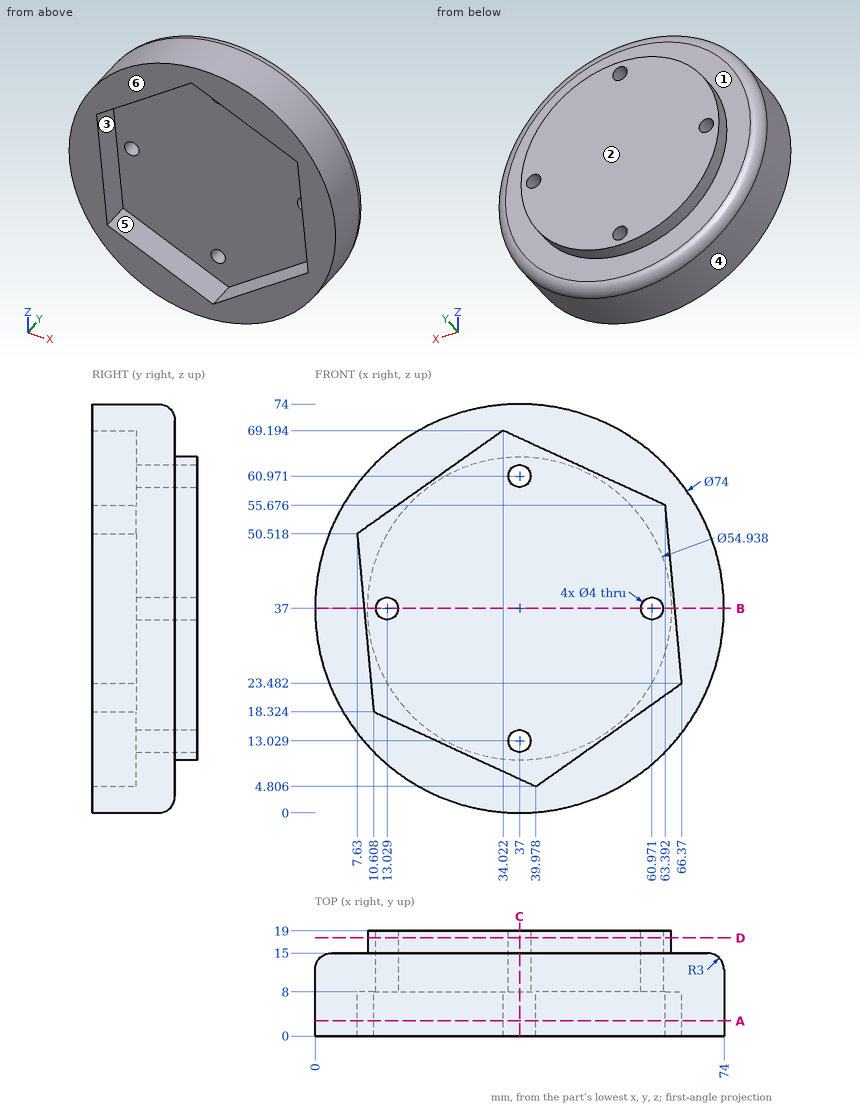
Check sheet for the drawn part. Datum: minimum x, y, z corner. Units: mm. A direction names the side the tool comes from. Round coordinates to 2 decimals unless told otherwise and drop trailing zeros. Order: outer loops, then holes, each group sorted by start corner. A loop starts at its lowest first (then second) coordinate and runs counter-clockwise, first axis right, second up.
(1) Go/stop test with flat-tipped pins: P1, Ø3, axis at y = 6, z = 16, coming from the -X side (1 decimal); P2, Ø10, axis at x = 11, y = 3, coming from the -Z side; P3, Ø17.5, axis at x = 25.5, z = 24, coming from the -Y side; P4, Ø3, axis at x = 13.029, z = 37, coming from the -Y side. Record where each tip stops, or that it passes through.
(2) Cross-section at D-D, the plane y = 17.75. Enter the section's corners in (x, z), and give its area (3 significant figures).
(3) Draft check along X on the marked faces 4, 5 and 6. Enter one of: pulls with the +X half, pulls with the -X half, needs draft (parallel to the pull), parting line crosses it, or undercut.
(4) Cross-section at B-B, the plane z = 37. Enter the section's corners in (x, y), and give its area (3 significant figures).
(5) Cross-section at A-A, the plane y = 2.75. Enter the section's corners in (x, z), and give its area (4 significant figures).
(6) Scan lines: probe 1 along Z at (x, y) = (37, 15.5); probe 2 along Z at (x, y) = (37, 14) (1 decimal); probe 3 along Y at (x, z) = (49, 57.5). Record each from-to range of solid material in increasing order.
(7) Cross-section at C-C, the plane x = 37. Enter the section's corners in (y, z), and give its area (3 significant figures).
(8) Access from +Z, -Z, +X, -X, +Y, -Y to the whole of each face (thin tool, end or side, straight path). Record for the marked faces 1, 2 and 3.
Check sheet entries:
1. P1: stops at x = 5.6
1. P2: stops at z = 6.54
1. P3: stops at y = 8
1. P4: passes through
2. outline: circle Ø54.94 at (37, 37); hole circle Ø4 at (13.03, 37); hole circle Ø4 at (37, 13.03); hole circle Ø4 at (37, 60.97); hole circle Ø4 at (60.97, 37)
2. area: 2,320 mm2
3. face 4: parting line crosses it
3. face 5: undercut
3. face 6: needs draft
4. outline: (0, 0) - (8.88, 0) - (8.88, 8) - (11.03, 8) - (11.03, 19) - (9.53, 19) - (9.53, 15) - (3, 15) arc R3 ccw to (0, 12) - close; (15.03, 8) - (58.97, 8) - (58.97, 19) - (15.03, 19) - close; (62.97, 8) - (65.12, 8) - (65.12, 0) - (74, 0) - (74, 12) arc R3 ccw to (71, 15) - (64.47, 15) - (64.47, 19) - (62.97, 19) - close
4. area: 788 mm2
5. outline: circle Ø74 at (37, 37); hole (7.63, 50.52) - (10.61, 18.32) - (39.98, 4.81) - (66.37, 23.48) - (63.39, 55.68) - (34.02, 69.19) - close
5. area: 1,585 mm2
6. probe 1: z = 9.53 to 11.03, 15.03 to 58.97, 62.97 to 64.47
6. probe 2: z = 0.8 to 11, 15 to 59, 63 to 73.2
6. probe 3: y = 8 to 19
7. outline: (0, 0) - (12, 0) arc R3 ccw to (15, 3) - (15, 9.53) - (19, 9.53) - (19, 11.03) - (8, 11.03) - (8, 6.18) - (0, 6.18) - close; (0, 67.82) - (8, 67.82) - (8, 62.97) - (19, 62.97) - (19, 64.47) - (15, 64.47) - (15, 71) arc R3 ccw to (12, 74) - (0, 74) - close; (8, 15.03) - (19, 15.03) - (19, 58.97) - (8, 58.97) - close
7. area: 745 mm2
8. face 1: +Y
8. face 2: +Z, -Z, +X, -X, +Y
8. face 3: -Y
